```python
from build123d import *

# Parameters (mm, degrees)
EXTRUDE_1_DEPTH     = 4
CUT_EXTRUDE_START   = -2
CUT_EXTRUDE_6_DEPTH = 3.5
EXTRUDE_2_DEPTH     = 0.5
SKETCH_8_W          = 4
SKETCH_8_H          = 3.5
CUT_EXTRUDE_7_DEPTH = 0.001


# Read off the part's stored shape, not the designer's step: the extrude step
with BuildPart() as part:
    # 草图4 → 凸台-拉伸1 (new body)
    with BuildSketch(Plane.XY):
        Polygon((17.75, -1.5), (8.5, -1.5), (4.5, 0), (4, 0), (0, 0), (-0.5, 0), (-4.5, -1.5), (-4.5, -3.5), (17.75, -3.5), align=None)
    extrude(amount=EXTRUDE_1_DEPTH)

    # 镜向1: part across plane


with BuildPart() as part_1:
    add(part.part)
    add(part.part.mirror(Plane.XY.offset(4)))

    # 镜向2: part across plane


with BuildPart() as part_2:
    add(part_1.part)
    add(part_1.part.mirror(Plane(origin=(17.75, 0, 4), x_dir=(0, 0, 1), z_dir=(1, 0, 0))))

    # 切除-拉伸6 outline → 切除-拉伸6 (cut)
    with BuildSketch(Plane(origin=(0, -1.5, 0), x_dir=(1, 0, 0), z_dir=(0, 1, 0)).offset(CUT_EXTRUDE_START)):
        Polygon((8.5, -4), (-4.5, -4), (-4.5, -8), (40, -8), (40, -4), (27, -4), (27, -2.5), (23, -2.5), (24.833333333, -5.5), (16.833333333, -5.5), (18.666666667, -2.5), (10.666666667, -2.5), (12.5, -5.5), (8.5, -5.5), align=None)
    extrude(amount=CUT_EXTRUDE_6_DEPTH, mode=Mode.SUBTRACT)

    # 草图7 → 凸台-拉伸2 (add)
    with BuildSketch(Plane(origin=(0, 0, 0), x_dir=(-1, 0, 0), z_dir=(0, 0, -1))):
        Polygon((0.5, 0), (-4.5, 0), (-8.5, -1.5), (-27, -1.5), (-31, 0), (-36, 0), (-40, -1.5), (-40, -3.5), (4.5, -3.5), (4.5, -1.5), align=None)
    extrude(amount=EXTRUDE_2_DEPTH)

    # 草图8 → 切除-拉伸7 (cut)
    with BuildSketch(Plane.XY.offset(4)):
        with Locations((33.5, -1.75)):
            Rectangle(SKETCH_8_W, SKETCH_8_H)
    extrude(amount=-CUT_EXTRUDE_7_DEPTH, mode=Mode.SUBTRACT)


solid = part_2.part
```
Check sheet for the modelled part. Datum: model origin and axes. Units: mm. A direction names the side the tool comes from. Round coordinates to 2 decimals unless told otherwise and drop trailing zeros. Order: outer loops, then holes, each group sorted by start corner. A loop starts at its lowest first (then second) coordinate and runs counter-clockwise, first axis right, second up.
1) Scan lines: line 1 (X direction, y = -1.85, z = 2.6); line 2 (Y direction, x = 13.5, z = 2.05); line 3 (Z direction, x = 15.5, y = -3.15). Record each from-to range of solid material in increasing order.
2) Tool access check on faces 5 (the flat face through (28.97, -0.76, 1.78)), 6 (the flat face through (38, -2, 4)), 7 (the flat face through (25, -3, 2.5)). Record the directions out of +Z, -Z, +X, -X, +Y, -Y that give a thin tool (end or side, any length) a straight path to the whole face; none if there is none.
3) Mould release check, pull along X, two halves, no side actions. Record for faces 1 (the flat face through (33, -2, 3.999)), 2 (the flat face through (23.904, -2.514, 3.979)), 3 (the flat face through (37.97, -0.74, 1.78)), 4 (the flat face through (11.57, -2.51, 3.98)): +X half, -X half, draft (parallel to the pull), parting line (faces both ways), or undercut.
4) Section check D-D (x = 17.5). Record the boundary of the cut face in (y, z).
5) Section check C-C (z = 4.4). Record the boundary of the cut face in (x, y).
6) Go/stop test with flat-tipped pins: pin 1 Ø3 at (x, z) = (14, 4.5) entering from +Y; pin 2 Ø3 at (x, z) = (15, 3) entering from +Y; pin 3 Ø1.8 at (x, y) = (29.5, -1.5) entering from +Z; pin 4 Ø1 at (x, y) = (14, -2.5) entering from +Z. Record where each tip stops, or that it passes through.
7) Section check A-A (z = 0.5). Record the boundary of the cut face in (x, y), and give its area (3 significant figures).
Result:
1. line 1: x = -4.5 to 10.73, 18.61 to 23.06, 27 to 40
1. line 2: y = -3.5 to -1.5
1. line 3: z = -0.5 to 2.5
2. face 5: +Z, -Z, +Y
2. face 6: +Z, +X, +Y, -Y
2. face 7: +Y, -Y
3. face 1: draft
3. face 2: undercut
3. face 3: +X half
3. face 4: undercut
4. outline: (-3.5, -0.5) - (-1.5, -0.5) - (-1.5, 2.5) - (-3.5, 2.5) - close; (-3.5, 4.41) - (-1.5, 4.41) - (-1.5, 5.5) - (-3.5, 5.5) - close
5. outline: (8.5, -3.5) - (11.83, -3.5) - (11.83, -1.5) - (8.5, -1.5) - close; (17.51, -3.5) - (24.16, -3.5) - (24.16, -1.5) - (17.51, -1.5) - close
6. pin 1: passes through
6. pin 2: stops at y = -1.5
6. pin 3: stops at z = 4
6. pin 4: stops at z = 2.5
7. outline: (-4.5, -3.5) - (40, -3.5) - (40, -1.5) - (36, 0) - (31, 0) - (27, -1.5) - (8.5, -1.5) - (4.5, 0) - (-0.5, 0) - (-4.5, -1.5) - close
7. area: 116 mm2
